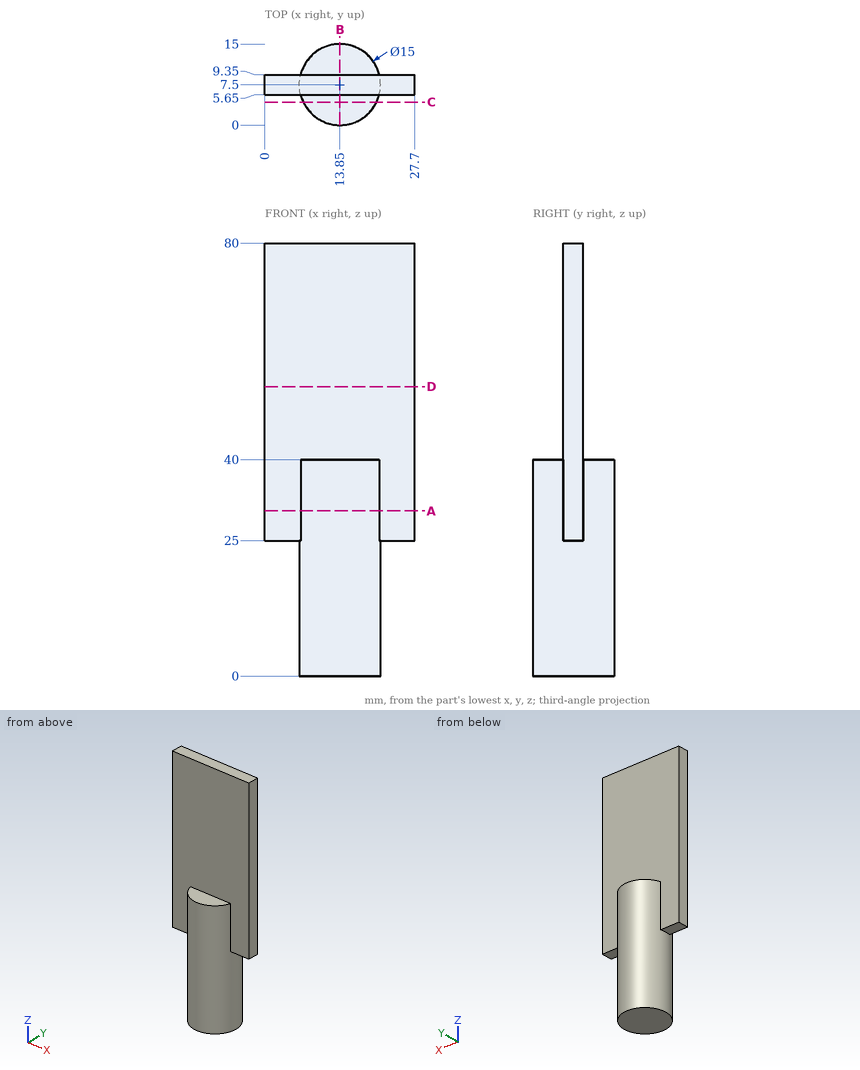
Part print with two shaded views. Sizes in mm from the minimum x, y, z corner. Round coordinates to 2 decimals unless told otherwise and drop trailing zeros. Order: outer loops, then holes, each group sorted by start corner. A loop starts at its lowest first (then second) coordinate and runs counter-clockwise, first axis right, second up. Notation, with made-up numbers: M -13,59 L -6,59 A18 ccw -6,68 Z; hole C 28.5,-15.75 d10. An arc over 180 degrees is marked long. Use CSV: the item, a comma, the result in double quotes.
Item 1: Saw through at A-A (z = 30.5). List the corners of the cut face in (x, y).
Worked answers:
outline,"M 0,5.65 L 6.58,5.65 A7.5 ccw 21.12,5.65 L 27.7,5.65 L 27.7,9.35 L 21.12,9.35 A7.5 ccw 6.58,9.35 L 0,9.35 Z"
Item 2: Saw through at C-C (y = 4.25). List the corners of the cut face in (x, z), plus the area to 3 significant figures.
Worked answers:
outline,"M 7.09,0 L 20.61,0 L 20.61,40 L 7.09,40 Z"
area,"541 mm²"
Item 3: Probe probe 1 along Y at (x, z) = (9.5, 54.5); probe 2 along Z at (x, y) = (12.5, 3.75); probe 3 along X at (y, z) = (2, 10.5). List the from-to ranges inside material, lowest first.
Worked answers:
probe 1,"5.65 to 9.35"
probe 2,"0 to 40"
probe 3,"8.75 to 18.95"
Item 4: Saw through at D-D (z = 53.5). List the corners of the cut face in (x, y).
Worked answers:
outline,"M 0,5.65 L 27.7,5.65 L 27.7,9.35 L 0,9.35 Z"
Item 5: Saw through at B-B (x = 13.85). List the corners of the cut face in (y, z), plus the area to 3 significant figures.
Worked answers:
outline,"M 0,0 L 15,0 L 15,40 L 9.35,40 L 9.35,80 L 5.65,80 L 5.65,40 L 0,40 Z"
area,"748 mm²"
Item 6: Pin check, flat tips, straight feed: pin 1 (1.9 mm diameter, centred on x = 24, y = 8, fed in from -Z); pin 2 (3 mm diameter, centred on x = 12.5, y = 11, fed in from +Z); pin 3 (14 mm diameter, centred on x = 13.5, z = 57, fed in from +Y). Stop position of each tip, or through.
Worked answers:
pin 1,"z = 25"
pin 2,"z = 40"
pin 3,"y = 9.35"
